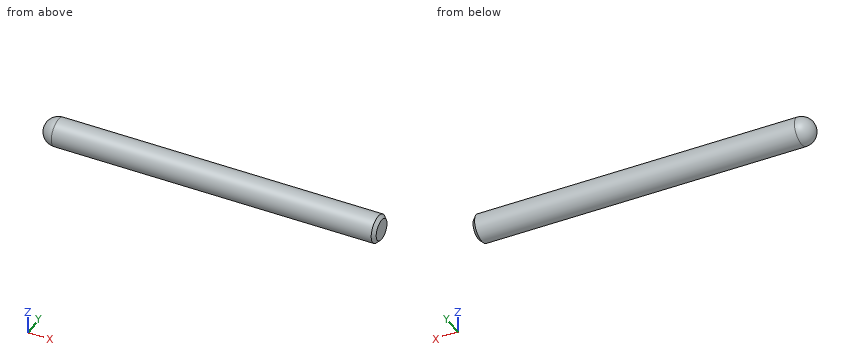
Autodesk Inventor part; units mm, degrees
ref_plane "YZ Plane" through (0, 0, 0) normal (1, 0, 0) x (0, 1, 0)
ref_plane "XZ Plane" through (0, 0, 0) normal (0, 1, 0) x (-1, 0, 0)
ref_plane "XY Plane" through (0, 0, 0) normal (0, 0, 1) x (1, 0, 0)
sketch "Sketch1" plane through (0, 0, 0) normal (1, 0, 0) x (0, 1, 0)
  circle A0 centre (0, 0) radius 3.175
  dimension "d0" = 6.35
extrude "Extrusion1" add sketch "Sketch1" along normal blind 77.7875
fillet "Fillet1" radius 3.175 1 edges at (0, -3.175, 0)
chamfer "Chamfer1" distance 0.762 angle 45 1 edges at (77.7875, -3.175, 0) measured on face at (77.7875, -0.5202, -0.7796)
thread "Thread1"
properties part number "lever arm"
Source: CAD feature listing. Evaluate the final solid. Frame: model axes, mm. Coordinates: 2 decimals unless noted, no trailing zeros. Write each loop counter-clockwise with the first axis right and the second up, starting at its lowest first coordinate (ties: lowest second). Pieces come first, ordered by that corner, then holes. Notation, with made-up numbers: M 10,85.25 L 14,85.25 A18 cw 14,114.25 Z; hole C 53.25,2 d1. An arc over 180 degrees is marked long. Use a Markdown table: item, result.
1) First-contact query: pin 1 Ø1.5 at (y, z) = (-2.5, 1.5) entering from -X. Flat tip, straight axial feed; report the tip coordinate or a pass-through.
Conclusion:
| item | result |
|---|---|
| pin 1 | stops at x = 0.85 |
2) Ray query, L1, parallel to Z at x = 35, y = 0.25; L2, parallel to Y at x = 41, z = -0.5. Return the intervals inside material, ascending.
Conclusion:
| item | result |
|---|---|
| L1 | z = -3.17 to 3.17 |
| L2 | y = -3.14 to 3.14 |
3) Section A-A, the plane x = 68.5. Output: boundary loops of the cut face in (y, z) (3 decimals).
Conclusion:
| item | result |
|---|---|
| outline | C 0,0 d6.35 |
